from build123d import *

# Parameters (mm, degrees)
CROQUIS1_W              = 150
CROQUIS1_H              = 101.6
SALIENTE_EXTRUIR1_DEPTH = 3.175
CROQUIS2_R              = 2
CROQUIS2_R_2            = 11
CROQUIS2_R_3            = 1.5
CROQUIS2_R_4            = 6.35
CORTAR_EXTRUIR1_DEPTH   = 91.807282197
REDONDEO1_R             = 6.35
CROQUIS3_R              = 1.5
CORTAR_EXTRUIR2_DEPTH   = 91.807282197
CORTAR_EXTRUIR3_START   = 3.175
CROQUIS4_R              = 12.5
CORTAR_EXTRUIR3_DEPTH   = 1.5
SALIENTE_EXTRUIR2_START = -6.35
CROQUIS5_W              = 150
CROQUIS5_H              = 6.35
SALIENTE_EXTRUIR2_DEPTH = 101.6
CROQUIS7_R              = 2
CORTAR_EXTRUIR5_DEPTH   = 161.109464508
CROQUIS9_R              = 2.5
CORTAR_EXTRUIR6_DEPTH   = 137.118330874
CHAFL_N1_SIZE           = 2.5
CROQUIS10_R             = 1.5
CORTAR_EXTRUIR7_DEPTH   = 157.157110389


with BuildPart() as part:
    # Croquis1 → Saliente-Extruir1 (new, symmetric)
    with BuildSketch(Plane(origin=(0, 0, 0), x_dir=(1, 0, 0), z_dir=(0, 1, 0))):
        Rectangle(CROQUIS1_W, CROQUIS1_H)
    extrude(amount=SALIENTE_EXTRUIR1_DEPTH, both=True)

    # Croquis2 → Cortar-Extruir1 (cut, through all)
    with BuildSketch(Plane(origin=(0, 3.175, 0), x_dir=(1, 0, 0), z_dir=(0, 1, 0))):
        with Locations(Location((67, 40.8, 0), (0, 0, 270))):
            Circle(CROQUIS2_R)
        with Locations(Location((67, -29.2, 0), (0, 0, 90))):
            Circle(CROQUIS2_R)
        with Locations(Location((-15, 5.8, 0), (0, 0, 270))):
            Circle(CROQUIS2_R_2)
        with Locations(Location((-67.25, 5.8, 0), (0, 0, 270))):
            Circle(CROQUIS2_R_3)
        with Locations(Location((31.9, 5.8, 0), (0, 0, 270))):
            Circle(CROQUIS2_R_4)
        with Locations((69.9, 5.8)):
            Circle(CROQUIS2_R_4)
    extrude(amount=-CORTAR_EXTRUIR1_DEPTH, mode=Mode.SUBTRACT)

    # Redondeo1
    redondeo1_edges = [part.edges().sort_by_distance(p)[0] for p in [
        (75, 0, -2.016813512),
        (75, 0, -9.583186488),
    ]]
    fillet(redondeo1_edges, radius=REDONDEO1_R)

    # Croquis3 → Cortar-Extruir2 (cut, through all)
    with BuildSketch(Plane(origin=(0, 3.175, 0), x_dir=(1, 0, 0), z_dir=(0, 1, 0))):
        with Locations(Location((-15, -9.2, 0), (0, 0, 270))):
            Circle(CROQUIS3_R)
        with Locations(Location((-15, -18.2, 0), (0, 0, 270))):
            Circle(CROQUIS3_R)
        with Locations(Location((-27.990381057, 13.3, 0), (0, 0, 270))):
            Circle(CROQUIS3_R)
        with Locations(Location((-35.784609691, 17.8, 0), (0, 0, 270))):
            Circle(CROQUIS3_R)
        with Locations(Location((-2.009618943, 13.3, 0), (0, 0, 270))):
            Circle(CROQUIS3_R)
        with Locations(Location((5.784609691, 17.8, 0), (0, 0, 270))):
            Circle(CROQUIS3_R)
    extrude(amount=-CORTAR_EXTRUIR2_DEPTH, mode=Mode.SUBTRACT)

    # Croquis4 → Cortar-Extruir3 (cut)
    with BuildSketch(Plane(origin=(0, 0, 0), x_dir=(1, 0, 0), z_dir=(0, 1, 0)).offset(CORTAR_EXTRUIR3_START)):
        with Locations(Location((-15, 5.8, 0), (0, 0, 270))):
            Circle(CROQUIS4_R)
    extrude(amount=-CORTAR_EXTRUIR3_DEPTH, mode=Mode.SUBTRACT)

    # Croquis5 → Saliente-Extruir2 (add)
    with BuildSketch(Plane.XZ.offset(3.175).offset(SALIENTE_EXTRUIR2_START)):
        with Locations((0, -47.625)):
            Rectangle(CROQUIS5_W, CROQUIS5_H)
    extrude(amount=SALIENTE_EXTRUIR2_DEPTH)

    # Croquis7 → Cortar-Extruir5 (cut, through all)
    with BuildSketch(Plane(origin=(0, 0, -50.8), x_dir=(-1, 0, 0), z_dir=(0, 0, -1))):
        with Locations((-60, -6.825)):
            Circle(CROQUIS7_R)
        with Locations((0, -6.825)):
            Circle(CROQUIS7_R)
        with Locations(Location((60, -6.825, 0), (0, 0, 180))):
            Circle(CROQUIS7_R)
        with Locations((60, -88.425)):
            Circle(CROQUIS7_R)
        with Locations(Location((0, -88.425, 0), (0, 0, 180))):
            Circle(CROQUIS7_R)
        with Locations(Location((-60, -88.425, 0), (0, 0, 180))):
            Circle(CROQUIS7_R)
        with Locations((-60, -37.625)):
            Circle(CROQUIS7_R)
        with Locations((0, -37.625)):
            Circle(CROQUIS7_R)
        with Locations(Location((60, -37.625, 0), (0, 0, 180))):
            Circle(CROQUIS7_R)
    extrude(amount=-CORTAR_EXTRUIR5_DEPTH, mode=Mode.SUBTRACT)

    # Croquis9 → Cortar-Extruir6 (cut, through all)
    with BuildSketch(Plane(origin=(0, 3.175, 0), x_dir=(1, 0, 0), z_dir=(0, 1, 0))):
        with Locations(Location((3.5, 5.8, 0), (0, 0, 270))):
            Circle(CROQUIS9_R)
        with Locations(Location((-33.5, 5.8, 0), (0, 0, 270))):
            Circle(CROQUIS9_R)
    extrude(amount=-CORTAR_EXTRUIR6_DEPTH, mode=Mode.SUBTRACT)

    # Chaflán1
    chafl_n1_edges = [part.edges().sort_by_distance(p)[0] for p in [
        (3.5, 3.175, -8.3),
        (-33.5, 3.175, -8.3),
    ]]
    chamfer(chafl_n1_edges, length=CHAFL_N1_SIZE)

    # Croquis10 → Cortar-Extruir7 (cut, through all)
    with BuildSketch(Plane.XY.offset(-44.45)):
        with Locations((15, -73.425)):
            Circle(CROQUIS10_R)
        with Locations(Location((-45, -73.425, 0), (0, 0, 180))):
            Circle(CROQUIS10_R)
    extrude(amount=-CORTAR_EXTRUIR7_DEPTH, mode=Mode.SUBTRACT)


solid = part.part
Verification items for the finished model (mm, model axes). A direction names the side the tool comes from. Coordinates: 2 decimals unless noted, no trailing zeros. Order: outer loops, then holes, each group sorted by start corner. A loop starts at its lowest first (then second) coordinate and runs counter-clockwise, first axis right, second up. Notation, with made-up numbers: M 25.25,50.5 L 64.25,50.5 A29 cw 64.25,86.5 Z; hole C 57,-24 d8. An arc over 180 degrees is marked long. Return JSON: item names as keys, results as strings.
1) Release check for a two-part mould opening along X. For faces 4 (the flat face through (-1, 3.175, -1)), 5 (the cylindrical face through (-0.43, -86.47, -47.67)), 6 (the flat face through (-75, -2, -22)) record: +X half, -X half, draft (parallel to the pull), parting line (faces both ways), or undercut.
Answer list:
{"face 4": "draft", "face 5": "undercut", "face 6": "-X half"}
2) Cross-section at C-C, the plane x = -11. Record the boundary of the cut face in (y, z) (3 decimals).
Answer list:
{"outline": "M -98.425,-50.8 L 3.175,-50.8 L 3.175,-17.643 L 1.675,-17.643 L 1.675,-16.047 L -3.175,-16.047 L -3.175,-44.45 L -98.425,-44.45 Z; M -3.175,4.447 L 1.675,4.447 L 1.675,6.043 L 3.175,6.043 L 3.175,50.8 L -3.175,50.8 Z"}
3) Cross-section at B-B, the plane y = -23. Record the boundary of the cut face in (x, z), and give its area (4 significant figures).
Answer list:
{"outline": "M -75,-50.8 L 75,-50.8 L 75,-44.45 L -75,-44.45 Z", "area": "952.5 mm2"}
4) Cross-section at D-D, the plane x = 54. Record the boundary of the cut face in (y, z) (3 decimals).
Answer list:
{"outline": "M -98.425,-50.8 L 3.175,-50.8 L 3.175,50.8 L -3.175,50.8 L -3.175,-44.45 L -98.425,-44.45 Z"}
5) Gauge pin test, flat ends, axial feed: pin 1 (4 mm diameter, centred on x = 15, y = -73.425, fed in from +Z); pin 2 (3.5 mm diameter, centred on x = 60, y = -6.825, fed in from -Z); pin 3 (1.5 mm diameter, centred on x = 4, z = 7.5, fed in from -Y) (3 decimals). Record the tip position at first contact, or that the pin passes through.
Answer list:
{"pin 1": "z = -44.45", "pin 2": "through", "pin 3": "y = -3.175"}
6) Cross-section at A-A, the plane x = 31.9. Record the boundary of the cut face in (y, z) (3 decimals).
Answer list:
{"outline": "M -98.425,-50.8 L 3.175,-50.8 L 3.175,-12.15 L -3.175,-12.15 L -3.175,-44.45 L -98.425,-44.45 Z; M -3.175,0.55 L 3.175,0.55 L 3.175,50.8 L -3.175,50.8 Z"}
7) Access from +Z, -Z, +X, -X, +Y, -Y to the whole of each face (thin tool, end or side, straight path). Record for faces 1 (the cylindrical face through (65.017, 0.044, 29.46)), 2 (the flat face through (-1, -50, -44.45)), 3 (the cylindrical face through (-27.203, 2.436, -8.51)).
Answer list:
{"face 1": "+Y, -Y", "face 2": "+Z, +X, -X, -Y", "face 3": "+Y"}
8) Thickness scan on L1, parallel to X at y = -0.75, z = -17.8; L2, parallel to Y at x = -60, z = -46 (3 decimals); L3, parallel to X at y = 0.05, z = -5.8. Record the ranges inside material, lowest first. Write a range as [from, to].
Answer list:
{"L1": "[-75, -37.28], [-34.28, 4.28], [7.28, 74.97]", "L2": "[-98.425, -90.425], [-86.425, -39.625], [-35.625, -8.825], [-4.825, 3.175]", "L3": "[-75, -68.75], [-65.75, -36], [-31, -26], [-4, 1], [6, 25.55], [38.25, 63.55]"}
